from build123d import *

# Parameters (mm, degrees)
SKETCH_W        = 34
SKETCH_H        = 34
PAD_DEPTH       = 80
POCKET_DEPTH    = 80
SKETCH002_R     = 3
POCKET001_DEPTH = 4
SKETCH003_R     = 3
POCKET002_DEPTH = 4
SKETCH004_R     = 4
POCKET003_DEPTH = 2
SKETCH005_R     = 4
POCKET004_DEPTH = 2
SKETCH006_W     = 6.4
SKETCH006_H     = 3
SKETCH006_W_2   = 8
SKETCH006_H_2   = 8
POCKET005_DEPTH = 16


with BuildPart() as part:
    # Sketch → Pad (new body)
    with BuildSketch(Plane.XY):
        with Locations((17, 17)):
            Rectangle(SKETCH_W, SKETCH_H)
    extrude(amount=PAD_DEPTH)

    # Sketch001 (on Face6 of Pad) → Pocket (cut)
    with BuildSketch(Plane.XY.offset(80)):
        Polygon((6.5, 27.5), (14, 27.5), (14, 23.5), (17, 21), (20, 23.5), (20, 27.5), (27.5, 27.5), (27.5, 19.5), (23.5, 19.5), (21, 17), (23.5, 14), (27.5, 14), (27.5, 6.5), (20, 6.5), (20, 10.5), (17, 13), (14, 10.5), (14, 6.5), (6.5, 6.5), (6.5, 14), (10.5, 14), (13, 17), (10.5, 19.5), (6.5, 19.5), align=None)
    extrude(amount=-POCKET_DEPTH, mode=Mode.SUBTRACT)

    # Sketch002 (on Face2 of Pocket) → Pocket001 (cut)
    with BuildSketch(Plane(origin=(0, 0, 0), x_dir=(0, -1, 0), z_dir=(-1, 0, 0))):
        with Locations((-17, 60)):
            Circle(SKETCH002_R)
        with Locations((-17, 20)):
            Circle(SKETCH002_R)
    extrude(amount=-POCKET001_DEPTH, mode=Mode.SUBTRACT)

    # Sketch003 (on Face3 of Pocket001) → Pocket002 (cut)
    with BuildSketch(Plane.YZ.offset(34)):
        with Locations((17, 60)):
            Circle(SKETCH003_R)
        with Locations((17, 20)):
            Circle(SKETCH003_R)
    extrude(amount=-POCKET002_DEPTH, mode=Mode.SUBTRACT)

    # Sketch004 (on Face1 of Pocket002) → Pocket003 (cut)
    with BuildSketch(Plane(origin=(0, 34, 0), x_dir=(-1, 0, 0), z_dir=(0, 1, 0))):
        with Locations((-27, 60)):
            Circle(SKETCH004_R)
        with Locations((-7, 60)):
            Circle(SKETCH004_R)
        with Locations((-27, 20)):
            Circle(SKETCH004_R)
        with Locations((-7, 20)):
            Circle(SKETCH004_R)
    extrude(amount=-POCKET003_DEPTH, mode=Mode.SUBTRACT)

    # Sketch005 (on Face10 of Pocket003) → Pocket004 (cut)
    with BuildSketch(Plane.XZ):
        with Locations((7, 60)):
            Circle(SKETCH005_R)
        with Locations((27, 60)):
            Circle(SKETCH005_R)
        with Locations((7, 20)):
            Circle(SKETCH005_R)
        with Locations((27, 20)):
            Circle(SKETCH005_R)
    extrude(amount=-POCKET004_DEPTH, mode=Mode.SUBTRACT)

    # Sketch006 (on Face4 of Pocket004) → Pocket005 (cut)
    with BuildSketch(Plane.XY.offset(80)):
        with Locations((17, 1.5)):
            Rectangle(SKETCH006_W, SKETCH006_H)
        with Locations((17, 10.5)):
            Rectangle(SKETCH006_W_2, SKETCH006_H_2)
    extrude(amount=-POCKET005_DEPTH, mode=Mode.SUBTRACT)


solid = part.part
Geometry check sheet. Reference: the model listing, model coordinates, mm. A direction names the side the tool comes from. Round coordinates to 2 decimals unless told otherwise and drop trailing zeros. Order: outer loops, then holes, each group sorted by start corner. A loop starts at its lowest first (then second) coordinate and runs counter-clockwise, first axis right, second up. Notation, with made-up numbers: (55, 73.25) - (103, 73.25) arc R21 cw to (103, 93.25) - close; hole circle Ø11 at (-7.75, 58.25). An arc over 180 degrees is marked (long way). One line per question, with ' | ' between items. Start each with the question number.
(1) Sectioned sample at B-B on x = 15.5. Record the cut outline in (y, z), and give its area (3 significant figures).
(2) Depth check by flat-ended pin: pin 1 Ø1.5 at (x, z) = (17.5, 54) entering from -Y; pin 2 Ø5.5 at (y, z) = (17, 60) entering from -X; pin 3 Ø4 at (x, z) = (28, 59) entering from +Y; pin 4 Ø1.8 at (x, y) = (16, 9) entering from +Z. Enter the tip coordinate at first touch or a pass-through.
(3) Sectioned sample at A-A on y = 12. Record the cut outline in (x, z), and give its area (3 significant figures).
(4) Sectioned sample at D-D on y = 16. Record the cut outline in (x, z).
(5) Thickness scan on L1, parallel to Z at x = 7, y = 33.1; L2, parallel to X at y = 10, z = 17; L3, parallel to Y at x = 20.5, z = 30.5. Record the ranges inside material, lowest first. Write a range as [from, to].
(6) Release check for a two-part mould opening along X. For faces 1 (the flat face through (17, 0, 39)), 2 (the cylindrical face through (6.479, 0.986, 23.966)), 3 (the flat face through (4, 17, 20)) record: released by +X, released by -X, zero draft, split by the parting line, or undercut.
(7) Sectioned sample at C-C on z = 41.5. Record the cut outline in (x, y), and give its area (3 significant figures).
(8) Access from +Z, -Z, +X, -X, +Y, -Y to the whole of each face (thin tool, end or side, straight path). Record for faces 4 (the cylindrical face through (24.05, 0.99, 22.7)), 5 (the flat face through (27, 32, 20)), 6 (the flat face through (26, 19.5, 41)), 7 (the cylindrical face through (32.03, 14.79, 62.03)), 8 (the cylindrical face through (2, 19.4, 18.2)).
Conclusion:
1) outline: (0, 0) - (11.75, 0) - (11.75, 64) - (6.5, 64) - (6.5, 80) - (3, 80) - (3, 64) - (0, 64) - close; (22.25, 0) - (34, 0) - (34, 80) - (22.25, 80) - close | area: 1,750 mm2
2) pin 1: stops at y = 0 | pin 2: stops at x = 4 | pin 3: stops at y = 32 | pin 4: stops at z = 64
3) outline: (0, 0) - (6.5, 0) - (6.5, 80) - (0, 80) - close; (15.8, 0) - (18.2, 0) - (18.2, 64) - (15.8, 64) - close; (27.5, 0) - (34, 0) - (34, 80) - (27.5, 80) - close | area: 1,190 mm2
4) outline: (0, 0) - (12.17, 0) - (12.17, 80) - (0, 80) - (0, 62.83) - (4, 62.83) - (4, 57.17) - (0, 57.17) - (0, 22.83) - (4, 22.83) - (4, 17.17) - (0, 17.17) - close; (21.83, 0) - (34, 0) - (34, 17.17) - (30, 17.17) - (30, 22.83) - (34, 22.83) - (34, 57.17) - (30, 57.17) - (30, 62.83) - (34, 62.83) - (34, 80) - (21.83, 80) - close
5) L1: z = [0, 16], [24, 56], [64, 80] | L2: x = [0, 6.5], [14, 20], [27.5, 34] | L3: y = [0, 6.5], [27.5, 34]
6) face 1: zero draft | face 2: undercut | face 3: released by -X
7) outline: (0, 0) - (34, 0) - (34, 34) - (0, 34) - close; hole (6.5, 6.5) - (14, 6.5) - (14, 10.5) - (17, 13) - (20, 10.5) - (20, 6.5) - (27.5, 6.5) - (27.5, 14) - (23.5, 14) - (21, 17) - (23.5, 19.5) - (27.5, 19.5) - (27.5, 27.5) - (20, 27.5) - (20, 23.5) - (17, 21) - (14, 23.5) - (14, 27.5) - (6.5, 27.5) - (6.5, 19.5) - (10.5, 19.5) - (13, 17) - (10.5, 14) - (6.5, 14) - close | area: 836 mm2
8) face 4: -Y | face 5: +Y | face 6: +Z, -Z | face 7: +X | face 8: -X
